Geometry: final body of the model. Coordinates: model frame, mm. A direction names the side the tool comes from. Give positions to 0.01 mm unless a question says otherwise; leave off trailing zeros. Write each loop counter-clockwise with the first axis right and the second up, starting at its lowest first coordinate (ties: lowest second). Pieces come first, ordered by that corner, then holes. Notation, with made-up numbers: (-16.75, 63) -> (5.25, 63) arc R34 ccw to (5.25, 98) -> close; hole circle Ø1 at (39, 8.5). An arc over 180 degrees is marked (long way). Answer in a Markdown table with one row per item. Add a question column.
Item 1: Draft query along X for faces 1 (the cylindrical face through (-13.227, -0.74, -23.109)), 2 (the flat face through (-17, 0, 6)), 3 (the cylindrical face through (-13.887, -1.972, -10.648)). Return one class per face: +X half, -X half, draft (parallel to the pull), parting line (faces both ways), or undercut.
Item 2: Access query for faces 4 (the cylindrical face through (-11.47, -0.74, 23.89)), 5 (the flat face through (-12.2, -1.5, -22.3)), 6 (the cylindrical face through (-5.598, -54.93, 42.634)), 7 (the flat face through (25.3, -1.5, 0.2)), 8 (the flat face through (-11, -1.5, 23)). Directions: +Z, -Z, +X, -X, +Y, -Y. A direction counts if a zero-diameter tool reaches every point of the face in a straight line with its end or side. Return the directions, or none.
Item 3: Section query A-A on y = -44.5. Output: boundary loops of the cut face in (x, z), plus the area to 3 significant figures.
Item 4: Section query B-B on y = -8. Output: boundary loops of the cut face in (x, z), plus the area to 3 significant figures.
Item 5: Material intervals for probe 1 along X at (y, z) = (-2.05, 0); probe 2 along Z at (x, y) = (0, -54); probe 3 along X at (y, z) = (-1, 0), sorted ascending. Write a range as from..to.
Item 6: First-contact query: P1, Ø1.7, axis at x = 24.5, z = 4.5, coming from the -Y side; P2, Ø6, axis at x = -29, y = -36.5, coming from the +Z side; P3, Ø1.5, axis at x = -16.5, z = -25.5, coming from the +Y side. Flat tips, straight axial feed; report the tip coordinate or a pass-through.
```python
from build123d import *

# Parameters (mm, degrees)
F0_R      = 17.5
F1_DEPTH  = 1.5
F2_R      = 25
F2_R_2    = 17.5
F3_DEPTH  = 2.5
F6_R      = 50
F5_R      = 25
F9_R      = 17.5
F8_R      = 43
F11_R     = 50
F11_R_2   = 43
F12_DEPTH = 10


with BuildPart() as f1:
    # F0 (on Front) → F1 (new body)
    with BuildSketch(Plane.XZ):
        with BuildLine():
            ThreePointArc((23.2602203248, -9.1630862947), (24.5612042469, -4.663394251), (25, 0))
            ThreePointArc((25, 0), (24.5634220452, 4.651698338), (23.2689362058, 9.1409303603))
            ThreePointArc((23.2689362058, 9.1409303603), (14.0797148585, 20.6582097362), (0, 25))
            ThreePointArc((0, 25), (-10.9669811321, 22.4660927811), (-19.7108172513, 15.3780259879))
            ThreePointArc((-19.7108172513, 15.3780259879), (-24.9555737451, 1.4897446272), (-21.4003229393, -12.9238608046))
            ThreePointArc((-21.4003229393, -12.9238608046), (-12.2862418967, -21.7726493578), (0, -25))
            ThreePointArc((0, -25), (14.0698763789, -20.6649117754), (23.2602203248, -9.1630862947))
        make_face()
        Circle(F0_R, mode=Mode.SUBTRACT)
        with BuildLine():
            ThreePointArc((23.2689362058, 9.1409303603), (24.5634220452, 4.651698338), (25, 0))
            ThreePointArc((25, 0), (24.5612042469, -4.663394251), (23.2602203248, -9.1630862947))
            Line((23.2602203248, -9.1630862947), (24.7313799339, -9.7426320713))
            ThreePointArc((24.7313799339, -9.7426320713), (26.6870958696, 0.0047625742), (24.9132933265, 9.7868968881))
            Line((24.9132933265, 9.7868968881), (23.2689362058, 9.1409303603))
        make_face()
        with BuildLine():
            ThreePointArc((-19.7108172513, 15.3780259879), (-10.9669811321, 22.4660927811), (0, 25))
            Line((0, 25), (0, 26.5))
            ThreePointArc((0, 26.5), (-11.625, 23.814058348), (-20.8934662864, 16.3007075472))
            Line((-20.8934662864, 16.3007075472), (-19.7108172513, 15.3780259879))
        make_face()
        with BuildLine():
            Line((0, -26.7237641467), (0, -25))
            ThreePointArc((0, -25), (-12.2862418967, -21.7726493578), (-21.4003229393, -12.9238608046))
            Line((-21.4003229393, -12.9238608046), (-22.6843423156, -13.6992924528))
            ThreePointArc((-22.6843423156, -13.6992924528), (-13.0611614327, -23.205443504), (0, -26.7237641467))
        make_face()
    extrude(amount=F1_DEPTH)

    # F2 (on face) → F3 (join)
    with BuildSketch(Plane.XZ.offset(1.5)):
        Circle(F2_R)
        Circle(F2_R_2, mode=Mode.SUBTRACT)
    extrude(amount=F3_DEPTH)

    # F6 (on offset) → F7 section 0
    with BuildSketch(Plane.XZ.offset(50)):
        Circle(F6_R)
    # F5 (on face) → F7 section 1
    with BuildSketch(Plane.XZ.offset(4)):
        Circle(F5_R)
    loft()

    # F9 (on face) → F10 section 0
    with BuildSketch(Plane(origin=(0, -4, 0), x_dir=(-1, 0, 0), z_dir=(0, 1, 0))):
        Circle(F9_R)
    # F8 (on face) → F10 section 1
    with BuildSketch(Plane.XZ.offset(50)):
        Circle(F8_R)
    loft(mode=Mode.SUBTRACT)

    # F11 (on face) → F12 (join)
    with BuildSketch(Plane.XZ.offset(50)):
        Circle(F11_R)
        Circle(F11_R_2, mode=Mode.SUBTRACT)
    extrude(amount=F12_DEPTH)


solid = f1.part
```
Findings below:
| question | item | result |
|---|---|---|
| 1 | face 1 | -X half |
| 1 | face 2 | draft |
| 1 | face 3 | undercut |
| 2 | face 4 | +Z, -X, +Y |
| 2 | face 5 | -Z, -X |
| 2 | face 6 | -Y |
| 2 | face 7 | +X |
| 2 | face 8 | +Z, -X |
| 3 | outline | circle Ø94.02 at (0, 0); hole circle Ø79.9 at (0, 0) |
| 3 | area | 1,930 mm^2 |
| 4 | outline | circle Ø54.35 at (0, 0); hole circle Ø39.43 at (0, 0) |
| 4 | area | 1,100 mm^2 |
| 5 | probe 1 | x = -25..-17.5, 17.5..25 |
| 5 | probe 2 | z = -50..-43, 43..50 |
| 5 | probe 3 | x = -25..-17.5, 17.5..26.69 |
| 6 | P1 | stops at y = -18.9 |
| 6 | P2 | stops at z = 34.61 |
| 6 | P3 | stops at y = -12.51 |
